Geometry check sheet. Reference: the model listing, model coordinates, mm. Coordinates: 2 decimals unless noted, no trailing zeros. Order: outer loops, then holes, each group sorted by start corner. A loop starts at its lowest first (then second) coordinate and runs counter-clockwise, first axis right, second up. Notation, with made-up numbers: M 38.5,47.25 L 79.5,47.25 A20 cw 79.5,83.25 Z; hole C -12,0 d8. An arc over 180 degrees is marked long. One line per item, written item: value. Start each with the question number.
1) Sectioned sample at C-C, the plane z = 0.95. Enter the section's corners in (x, y), then the cut area to 3 significant figures.
2) Sectioned sample at A-A, the plane x = -34.5. Enter the section's corners in (y, z).
3) Go/stop test with a flat-tipped pin: P1, Ø10, axis at x = 100, y = -108, coming from the -Z side. Record where the tip stops, or that it passes through.
4) Thickness scan on L1, parallel to Y at x = 21.5, z = 4.2; L2, parallel to X at y = -173, z = 4.15. Record the ranges inside material, lowest first. Write a range as from..to.
5) Sectioned sample at B-B, the plane y = -153.5. Enter the section's corners in (x, z).
Autodesk Inventor part; units mm, degrees
ref_plane "YZ Plane" through (0, 0, 0) normal (1, 0, 0) x (0, 1, 0)
ref_plane "XZ Plane" through (0, 0, 0) normal (0, 1, 0) x (-1, 0, 0)
ref_plane "XY Plane" through (0, 0, 0) normal (0, 0, 1) x (1, 0, 0)
sketch "Sketch1" plane through (0, 0, 0) normal (0, 0, 1) x (1, 0, 0)
  line L0 (-225, -325) -> (225, -325)
  line L1 (225, -325) -> (225, 325)
  line L2 (225, 325) -> (-225, 325)
  line L3 (-225, 325) -> (-225, -325)
  line L4 (-225, -325) -> (225, 325) construction
  line L5 (225, -325) -> (-225, 325) construction
  line L6 (-195, -185) -> (195, -185)
  line L7 (195, -185) -> (195, -100)
  line L8 (195, -100) -> (-195, -100)
  line L9 (-195, -100) -> (-195, -185)
  line L10 (-195, -185) -> (195, -100) construction
  line L11 (195, -185) -> (-195, -100) construction
  point P0 (0, 0)
  point P1 (0, -142.5)
  dimension "d0" = 450
  dimension "d1" = 650
  dimension "d4" = 140
  dimension "d5" = 225
  dimension "d6" = 390
extrude "Extrusion1" add sketch "Sketch1" along normal blind 5
properties part number "Foam Sheet Front" material "PVC-Piping"
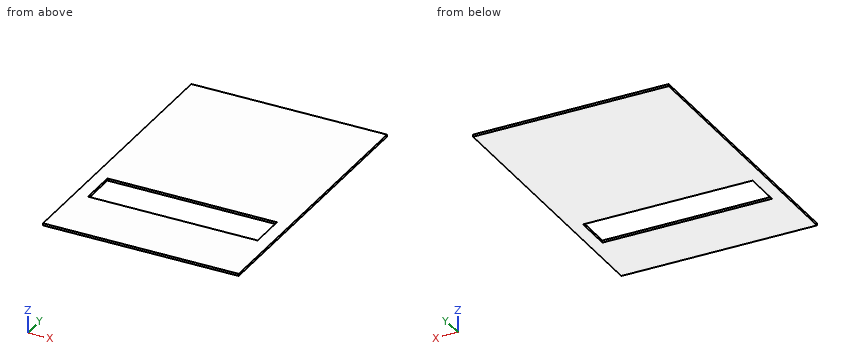
Final values:
1. outline: M -225,-325 L 225,-325 L 225,325 L -225,325 Z; hole M -195,-185 L 195,-185 L 195,-100 L -195,-100 Z
1. area: 259,000 mm^2
2. outline: M -325,0 L -185,0 L -185,5 L -325,5 Z; M -100,0 L 325,0 L 325,5 L -100,5 Z
3. P1: passes through
4. L1: y = -325..-185, -100..325
4. L2: x = -225..-195, 195..225
5. outline: M -225,0 L -195,0 L -195,5 L -225,5 Z; M 195,0 L 225,0 L 225,5 L 195,5 Z
